Build history of the part. All positions in model axes, mm. A direction names the side the tool comes from. Give positions to 0.01 mm unless a question says otherwise; leave off trailing zeros. Order: outer loops, then holes, each group sorted by start corner. A loop starts at its lowest first (then second) coordinate and runs counter-clockwise, first axis right, second up. Notation, with made-up numbers: (74, 0.5) -> (108, 0.5) arc R34 ccw to (108, 31.5) -> close; hole circle Ø9 at (-34, -15.75). An arc over 180 degrees is marked (long way). One line per question, with ' | ' between items. Start each with the question number.
(1) Drill centre lines: L1, parallel to Y at x = -6.5, z = 0; L2, parallel to Z at x = -11, y = -14; L3, parallel to X at y = 17, z = -29. Where is each one in solid material? Low to high. Write a range as from..to.
(2) Pull direction Y, two halves, no side cores. Call faces 1 (the face through (0, -10.2, -0.1)), 2 (the face through (54, 8, 0)), 3 (the face through (-9, 47, 0)): +Y half, -Y half, draft (parallel to the pull), parting line (faces both ways), or undercut.
(3) Cut at A-A (z = -26.5). Give the cut face in (x, y), then the cut area to 3 significant figures.
(4) Cut at C-C (x = -7). Give the number of separate pieces and of enclosed holes in the cut face, then the cut area to 3 significant figures.
(5) Cut at B-B (y = 0). Give the cut face in (x, z).
(6) Which spindle directions (+Z, -Z, +X, -X, +Y, -Y) get a long thin tool onto all of the face, cutting with end or side? Do faces 4 (the face through (47, -8.2, -1.5)), 5 (the face through (53, -10, 0)), 6 (the face through (-9.07, 22.87, 35.64)). Say none if no direction does.
(7) Pin check, flat tips, straight feed: pin 1 Ø3 at (x, z) = (53, 0) entering from +Y; pin 2 Ø7 at (y, z) = (-31.11, 31.11) entering from -X; pin 3 Ø1 at (x, y) = (-1.5, -11) entering from +Z; pin 4 Ø5 at (y, z) = (-18, -34) entering from +X. Stop position of each tip, or through.
from build123d import *

# Parameters (mm, degrees)
ENL_V_MAT_EXTRU_1_REACH      = 102.291
ESQUISSE2_R                  = 3
TROU_TARAUD_M61_D            = 5
R_P_TITION_CIRCULAIRE1_COUNT = 3
ENL_V_MAT_EXTRU_4_REACH      = 102.291
ESQUISSE4_W                  = 4
ESQUISSE4_H                  = 4.231945228


with BuildPart() as part:
    # Esquisse1 → Révolution1 (revolve)
    with BuildSketch(Plane.XY, mode=Mode.PRIVATE) as r_volution1_sk:
        with BuildLine():
            Line((-14, 0), (-14, 49))
            Line((-14, 49), (-4, 49))
            Line((-4, 49), (-4, 14.5))
            ThreePointArc((-4, 14.5), (-3.414213562, 13.085786438), (-2, 12.5))
            Line((-2, 12.5), (0, 12.5))
            Line((0, 12.5), (0, 10))
            Line((0, 10), (47, 10))
            Line((47, 10), (47, 8.12772302))
            Line((47, 8.12772302), (48.5, 8.12772302))
            Line((48.5, 8.12772302), (48.5, 10))
            Line((48.5, 10), (57, 10))
            Line((57, 10), (58.5, 8.5))
            Line((58.5, 8.5), (58.5, 0))
            Line((58.5, 0), (-14, 0))
        make_face()
    revolve(r_volution1_sk.sketch.rotate(Axis((-18.286431075, 0, 0), (1, 0, 0)), 90), axis=Axis((-18.286431075, 0, 0), (1, 0, 0)))

    # Esquisse2 → Enlèv. mat.-Extru.1 (cut, up to next)
    with BuildSketch(Plane.ZY.offset(14), mode=Mode.PRIVATE) as enl_v_mat_extru_1_sk1:
        with Locations((0, -30)):
            Circle(ESQUISSE2_R)
    enl_v_mat_extru_1_tool1 = extrude(enl_v_mat_extru_1_sk1.sketch, amount=-ENL_V_MAT_EXTRU_1_REACH, mode=Mode.PRIVATE) & part.part
    # Esquisse2 → Enlèv. mat.-Extru.1 (cut, up to next)
    with BuildSketch(Plane.ZY.offset(14), mode=Mode.PRIVATE) as enl_v_mat_extru_1_sk2:
        with Locations((-21.213203436, 21.213203436)):
            Circle(ESQUISSE2_R)
    enl_v_mat_extru_1_tool2 = extrude(enl_v_mat_extru_1_sk2.sketch, amount=-ENL_V_MAT_EXTRU_1_REACH, mode=Mode.PRIVATE) & part.part
    # Esquisse2 → Enlèv. mat.-Extru.1 (cut, up to next)
    with BuildSketch(Plane.ZY.offset(14), mode=Mode.PRIVATE) as enl_v_mat_extru_1_sk3:
        with Locations((0, 44)):
            Circle(ESQUISSE2_R)
    enl_v_mat_extru_1_tool3 = extrude(enl_v_mat_extru_1_sk3.sketch, amount=-ENL_V_MAT_EXTRU_1_REACH, mode=Mode.PRIVATE) & part.part
    # Esquisse2 → Enlèv. mat.-Extru.1 (cut, up to next)
    with BuildSketch(Plane.ZY.offset(14), mode=Mode.PRIVATE) as enl_v_mat_extru_1_sk4:
        with Locations((31.112698372, -31.112698372)):
            Circle(ESQUISSE2_R)
    enl_v_mat_extru_1_tool4 = extrude(enl_v_mat_extru_1_sk4.sketch, amount=-ENL_V_MAT_EXTRU_1_REACH, mode=Mode.PRIVATE) & part.part
    add(enl_v_mat_extru_1_tool1.solids().sort_by_distance((-14, -30, 0))[0], mode=Mode.SUBTRACT)
    add(enl_v_mat_extru_1_tool2.solids().sort_by_distance((-14, 21.213203, -21.213203))[0], mode=Mode.SUBTRACT)
    add(enl_v_mat_extru_1_tool3.solids().sort_by_distance((-14, 44, 0))[0], mode=Mode.SUBTRACT)
    add(enl_v_mat_extru_1_tool4.solids().sort_by_distance((-14, -31.112698, 31.112698))[0], mode=Mode.SUBTRACT)

    # Trou taraudé M61 (through all)
    with Locations(Plane(origin=(-4, 29.732137495, 0), x_dir=(0, 0, 1), z_dir=(1, 0, 0))):
        with Locations((0, 0), (0, 73.549942095)):
            trou_taraud_m61 = Hole(TROU_TARAUD_M61_D / 2)

    # Répétition circulaire1: Trou taraudé M61 ×3 about axis
    r_p_tition_circulaire1_axis = Axis((0, 0, 0), (1, 0, 0))
    for i in range(1, R_P_TITION_CIRCULAIRE1_COUNT):
        add(trou_taraud_m61.rotate(r_p_tition_circulaire1_axis, i * 360 / R_P_TITION_CIRCULAIRE1_COUNT), mode=Mode.SUBTRACT)

    # Enlèv. mat.-Extru.4: up to this face of the body (flat: up to its plane)
    enl_v_mat_extru_4_end = Plane(part.part.faces().sort_by_distance((48.5, 0, -8.410565733))[0])
    # Esquisse4 → Enlèv. mat.-Extru.4 (cut, up to the picked face)
    with BuildSketch(Plane(origin=(58.5, 0, 0), x_dir=(0, 0, -1), z_dir=(1, 0, 0)), mode=Mode.PRIVATE) as enl_v_mat_extru_4_sk1:
        with Locations((0, 10.115972614)):
            Rectangle(ESQUISSE4_W, ESQUISSE4_H)
    enl_v_mat_extru_4_tool1 = split(extrude(enl_v_mat_extru_4_sk1.sketch, amount=-ENL_V_MAT_EXTRU_4_REACH, mode=Mode.PRIVATE), bisect_by=enl_v_mat_extru_4_end, keep=Keep.BOTH, mode=Mode.PRIVATE)
    add(enl_v_mat_extru_4_tool1.solids().sort_by(Axis((58.5, 10.115973, 0), (-1, 0, 0)))[0], mode=Mode.SUBTRACT)


solid = part.part
Result set:
1) L1: y = -49..-46.32, -41.32..-33, -27..27.23, 32.23..41, 47..49 | L2: z = -46.96..-28.09, -23.4..23.4, 28.09..46.96 | L3: x = -14..-4
2) face 1: draft | face 2: +Y half | face 3: undercut
3) outline: (-14, -41.22) -> (-4, -41.22) -> (-4, -17.25) -> (-14, -17.25) -> close; (-14, -12.48) -> (-4, -12.48) -> (-4, 41.22) -> (-14, 41.22) -> close | area: 777 mm2
4) separate pieces: 1 | enclosed holes: 10 | area: 7,310 mm2
5) outline: (-14, -49) -> (-4, -49) -> (-4, -14.5) arc R2 cw to (-2, -12.5) -> (0, -12.5) -> (0, -10) -> (47, -10) -> (47, -8.13) -> (48.5, -8.13) -> (48.5, -10) -> (57, -10) -> (58.5, -8.5) -> (58.5, 8.5) -> (57, 10) -> (48.5, 10) -> (48.5, 8.13) -> (47, 8.13) -> (47, 10) -> (0, 10) -> (0, 12.5) -> (-2, 12.5) arc R2 cw to (-4, 14.5) -> (-4, 49) -> (-14, 49) -> close
6) face 4: none | face 5: +X | face 6: +X, -X
7) pin 1: stops at y = 8 | pin 2: stops at x = -14 | pin 3: stops at z = 6.78 | pin 4: stops at x = -4
